```python
from build123d import *

# Parameters (mm, degrees)
SKETCH_1_W                = 240
SKETCH_1_H                = 215
EXTRUDE_1_DEPTH           = 314
SKETCH_2_W                = 93.930111424
SKETCH_2_H                = 33.454560233
SKETCH_2_W_2              = 70
SKETCH_2_H_2              = 30.443707166
CUT_EXTRUDE_1_DEPTH       = 353.91960841
CHAMFER_1_SIZE            = 2
SKETCH_3_R                = 6
EXTRUDE_2_DEPTH           = 15
SKETCH_4_R                = 3
CUT_EXTRUDE_2_DEPTH       = 354.844951921
SKETCH_5_R                = 11
EXTRUDE_3_DEPTH           = 15
EXTRUDE_3_DRAFT           = 10
EXTRUDE_3_PROFILE_2_DEPTH = 15
EXTRUDE_3_PROFILE_2_DRAFT = 10
CHAMFER_2_SIZE            = 1


with BuildPart() as part:
    # 草图1 → 凸台-拉伸1 (new body)
    with BuildSketch(Plane.XY):
        Rectangle(SKETCH_1_W, SKETCH_1_H)
    extrude(amount=EXTRUDE_1_DEPTH)

    # 草图2 → 切除-拉伸1 (cut, through all)
    with BuildSketch(Plane.XY.offset(314)):
        with Locations((-96.965055712, 112.227280116)):
            Rectangle(SKETCH_2_W, SKETCH_2_H)
        with Locations((85, 110.721853583)):
            Rectangle(SKETCH_2_W_2, SKETCH_2_H_2)
    extrude(amount=-CUT_EXTRUDE_1_DEPTH, mode=Mode.SUBTRACT)

    # 倒角1
    chamfer_1_edges = [part.edges().sort_by_distance(p)[0] for p in [
        (-50, 107.5, 157),
        (-120, 95.5, 157),
        (50, 107.5, 157),
        (120, 95.5, 157),
    ]]
    chamfer(chamfer_1_edges, length=CHAMFER_1_SIZE)

    # 草图3 → 凸台-拉伸2 (add)
    with BuildSketch(Plane(origin=(0, 95.5, 0), x_dir=(1, 0, 0), z_dir=(0, 1, 0))):
        with Locations(Location((-100, -70, 0), (0, 0, 90))):
            Circle(SKETCH_3_R)
        with Locations(Location((-100, -244, 0), (0, 0, 90))):
            Circle(SKETCH_3_R)
    extrude_2 = extrude(amount=EXTRUDE_2_DEPTH)

    # 草图4 → 切除-拉伸2 (cut, through all)
    with BuildSketch(Plane.XY.offset(314)):
        with Locations((-100, 105.5)):
            Circle(SKETCH_4_R)
    cut_extrude_2 = extrude(amount=-CUT_EXTRUDE_2_DEPTH, mode=Mode.SUBTRACT)


with BuildPart() as extrude_3_tool:
    # 草图5 → 凸台-拉伸3 (with draft: the straight prism first)
    with BuildSketch(Plane(origin=(0, 107.5, 0), x_dir=(1, 0, 0), z_dir=(0, 1, 0))):
        with Locations((0, -45)):
            Circle(SKETCH_5_R)
    extrude(amount=EXTRUDE_3_DEPTH)
    # 凸台-拉伸3: the draft: its side faces are tilted about the plane it starts from
    extrude_3_sides = [extrude_3_tool.faces().sort_by_distance(p)[0] for p in [
        (-11, 115, 45),
    ]]
    draft(extrude_3_sides, Plane(origin=(0, 107.5, 0), x_dir=(1, 0, 0), z_dir=(0, 1, 0)), EXTRUDE_3_DRAFT)


with BuildPart() as part_1:
    add(part.part)

    # 凸台-拉伸3: add extrude_3_tool
    add(extrude_3_tool.part)


with BuildPart() as extrude_3_profile_2_tool:
    # 草图5 → 凸台-拉伸3 profile 2 (with draft: the straight prism first)
    with BuildSketch(Plane(origin=(0, 107.5, 0), x_dir=(1, 0, 0), z_dir=(0, 1, 0))):
        with Locations((0, -269)):
            Circle(SKETCH_5_R)
    extrude(amount=EXTRUDE_3_PROFILE_2_DEPTH)
    # 凸台-拉伸3 profile 2: the draft: its side faces are tilted about the plane it starts from
    extrude_3_profile_2_sides = [extrude_3_profile_2_tool.faces().sort_by_distance(p)[0] for p in [
        (-11, 115, 269),
    ]]
    draft(extrude_3_profile_2_sides, Plane(origin=(0, 107.5, 0), x_dir=(1, 0, 0), z_dir=(0, 1, 0)), EXTRUDE_3_PROFILE_2_DRAFT)


with BuildPart() as part_2:
    add(part_1.part)

    # 凸台-拉伸3 profile 2: add extrude_3_profile_2_tool
    add(extrude_3_profile_2_tool.part)

    # 镜向1: 凸台-拉伸2, 切除-拉伸2 across plane
    add(extrude_2.mirror(Plane(origin=(0, 0, 0), x_dir=(0, 0, 1), z_dir=(1, 0, 0))))
    add(cut_extrude_2.mirror(Plane(origin=(0, 0, 0), x_dir=(0, 0, 1), z_dir=(1, 0, 0))), mode=Mode.SUBTRACT)

    # 倒角2
    chamfer_2_edges = [part_2.edges().sort_by_distance(p)[0] for p in [
        (0, -107.5, 314),
        (-84, 95.5, 0),
        (-50, 100.5, 314),
        (-50, 100.5, 0),
        (50, 100.5, 0),
        (84, 95.5, 314),
        (84, 95.5, 0),
        (120, -7, 314),
        (0, -107.5, 0),
        (-120, -7, 314),
        (-120, -7, 0),
        (0, 107.5, 0),
        (-49, 106.5, 0),
        (49, 106.5, 0),
        (119, 94.5, 0),
        (-119, 94.5, 0),
        (-84, 95.5, 314),
        (120, -7, 0),
        (50, 100.5, 314),
        (0, 107.5, 314),
        (-49, 106.5, 314),
        (49, 106.5, 314),
        (119, 94.5, 314),
        (-119, 94.5, 314),
    ]]
    chamfer(chamfer_2_edges, length=CHAMFER_2_SIZE)


solid = part_2.part
```
Input: part model. Units: mm. Frame: model coordinates. A direction names the side the tool comes from. Coordinates: 2 decimals unless noted, no trailing zeros. Loops run counter-clockwise (first coordinate to the right, second up) from the corner with the lowest first, then second, coordinate; pieces in that order, holes last. Notation, with made-up numbers: M 22.25,-19.5 L 44.25,-19.5 A15 cw 44.25,0.5 Z; hole C -16.5,20.25 d8. An arc over 180 degrees is marked long. Use a Markdown table: item, result. Add a question column.
1) Pin query (flat end, axial travel): P1, Ø13, axis at x = -102, z = 244.5, coming from the +Y side; P2, Ø2, axis at y = 96, z = 82, coming from the +X side; P3, Ø7, axis at x = 100, y = 105.5, coming from the -Z side. Return the tip coordinate at first contact, or that it passes through.
2) Section A-A, the plane z = 200. Return the cut outline in (x, y), plus the area to 3 significant figures.
3) Section B-B, the plane x = 76. Return the cut outline in (y, z), plus the area to 3 significant figures.
4) Draft query along Z for faces 1 (the flat face through (-120, -8, 155)), 2 (the flat face through (-2, 1, 0)), 3 (the cylindrical face through (-96.35, 102.9, 248.76)). Return one class per face: +Z half, -Z half, draft (parallel to the pull), parting line (faces both ways), or undercut.
5) Section C-C, the plane z = 269. Return the cut outline in (x, y).
6) Section D-D, the plane x = 0. Return the cut outline in (y, z).
7) Line query: L1, parallel to X at y = 105.5, z = 244.5; L2, parallel to X at y = 105.5, z = 69; L3, parallel to Y at x = 100, z = 242. Output: solid intervals per line, ascending. Write a range as from..to.
8) Set-up query: faces 4 (the flat face through (120, -8, 155)), 5 (the cylindrical face through (-96.35, 102.9, 74.76)). Return all of +Z, -Z, +X, -X, +Y, -Y with unobstructed straight access to the full face (end or side cutting, diameter ignored); none if empty.
Answer below:
| question | item | result |
|---|---|---|
| 1 | P1 | y = 110.5 |
| 1 | P2 | x = 118.5 |
| 1 | P3 | z = 64 |
| 2 | outline | M -120,-107.5 L 120,-107.5 L 120,93.5 L 118,95.5 L 50,95.5 L 50,105.5 L 48,107.5 L -48,107.5 L -50,105.5 L -50,95.5 L -118,95.5 L -120,93.5 Z |
| 2 | area | 49,900 mm2 |
| 3 | outline | M -107.5,1 L -106.5,0 L 94.5,0 L 95.5,1 L 95.5,313 L 94.5,314 L -106.5,314 L -107.5,313 Z |
| 3 | area | 63,700 mm2 |
| 4 | face 1 | draft |
| 4 | face 2 | -Z half |
| 4 | face 3 | undercut |
| 5 | outline | M -120,-107.5 L 120,-107.5 L 120,93.5 L 118,95.5 L 50,95.5 L 50,105.5 L 48,107.5 L 11,107.5 L 8.36,122.5 L -8.36,122.5 L -11,107.5 L -48,107.5 L -50,105.5 L -50,95.5 L -118,95.5 L -120,93.5 Z |
| 6 | outline | M -107.5,1 L -106.5,0 L 106.5,0 L 107.5,1 L 107.5,34 L 122.5,36.64 L 122.5,53.36 L 107.5,56 L 107.5,258 L 122.5,260.64 L 122.5,277.36 L 107.5,280 L 107.5,313 L 106.5,314 L -106.5,314 L -107.5,313 Z |
| 7 | L1 | -105.98..-103, -97..-94.02, -50..50, 94.02..97, 103..105.98 |
| 7 | L2 | -105.92..-103, -97..-94.08, -50..50, 94.08..97, 103..105.92 |
| 7 | L3 | -107.5..102.5, 108.5..110.5 |
| 8 | face 4 | +Z, -Z, +X, +Y, -Y |
| 8 | face 5 | +Y |
